Source: CAD feature listing. Evaluate the final solid. Frame: model axes, mm. Round coordinates to 2 decimals unless told otherwise and drop trailing zeros. Use one line per item in the form item = value. Start each with the question number.
Q1. Pin query (flat end, axial travel): pin 1 Ø5.5 at (x, y) = (98.41, 45.9) entering from +Z. Return the tip coordinate at first contact, or that it passes through.
Q2. Ray query, line 1 (X direction, y = 45.75, z = 3.9); line 2 (X direction, y = 47, z = 2.6); line 3 (Y direction, x = 99, z = 2.1). Return the intervals inside material, ascending. Write a range as [from, to].
Q3. Draft query along Y for faces 1 (the flat face through (104.756, 45, 2)), 2 (the cylindrical face through (97.61, 47.43, 2.35)), 3 (the cylindrical face through (-26.27, 51.48, 2.41)). Return one class per face: released by +Y, released by -Y, zero draft, split by the parting line, or undercut.
from build123d import *

# Parameters (mm, degrees)
SKETCH1_W           = 131.7498
SKETCH1_H           = 12.7
SKETCH1_R           = 1.7272
BOSS_EXTRUDE1_DEPTH = 4.7625
FILLET1_R           = 2.54


with BuildPart() as part:
    # Sketch1 → Boss-Extrude1 (new body)
    with BuildSketch(Plane.XY):
        with Locations((38.881044974, 45.895610345)):
            Rectangle(SKETCH1_W, SKETCH1_H)
        with Locations(Location((-20.643855026, 45.895610345, 0), (0, 0, 180))):
            Circle(SKETCH1_R, mode=Mode.SUBTRACT)
        with Locations(Location((98.405944974, 45.895610345, 0), (0, 0, 180))):
            Circle(SKETCH1_R, mode=Mode.SUBTRACT)
    extrude(amount=BOSS_EXTRUDE1_DEPTH)

    # Fillet1
    fillet1_edges = [part.edges().sort_by_distance(p)[0] for p in [
        (-26.993855026, 52.245610345, 2.38125),
        (104.755944974, 52.245610345, 2.38125),
    ]]
    fillet(fillet1_edges, radius=FILLET1_R)


solid = part.part
Completed:
q1.pin_1 = 4.76
q2.line_1 = [-26.99, -22.36], [-18.92, 96.68], [100.13, 104.76]
q2.line_2 = [-26.99, -21.97], [-19.32, 97.08], [99.73, 104.76]
q2.line_3 = [39.55, 44.27], [47.52, 52.25]
q3.face_1 = zero draft
q3.face_2 = undercut
q3.face_3 = released by +Y
